Geometry: final body of the model. Coordinates: model frame, mm. Give positions to 0.01 mm unless a question says otherwise; leave off trailing zeros. Write each loop counter-clockwise with the first axis right and the second up, starting at its lowest first coordinate (ties: lowest second). Pieces come first, ordered by that corner, then holes.
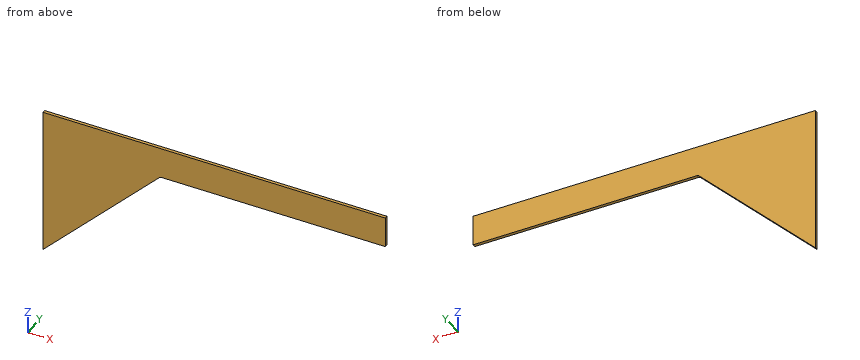
from build123d import *

# Parameters (mm, degrees)
BOSS_EXTRUDE1_DEPTH = 3.175
FILLET1_R           = 2.54


with BuildPart() as part:
    # Sketch1 → Boss-Extrude1 (new body)
    with BuildSketch(Plane(origin=(0, 0, 0), x_dir=(1, 0, 0), z_dir=(0, 1, 0))):
        Polygon((152.4, 0), (0, 0), (0, 152.4), align=None)
        Polygon((120.65, 31.75), (152.4, 0), (352.425, 0), (352.425, 31.75), (121.965128061, 31.75), align=None)
    extrude(amount=BOSS_EXTRUDE1_DEPTH)

    # Fillet1
    fillet1_edges = [part.edges().sort_by_distance(p)[0] for p in [
        (120.65, 1.5875, -31.75),
    ]]
    fillet(fillet1_edges, radius=FILLET1_R)


solid = part.part
Q1. Ray query, line 1 along Z through (x, y) = (336, 1.4); line 2 along X through (y, z) = (0.85, -104); line 3 along Z through (x, y) = (77, 1.7). Return the intervals inside material, ascending.
Filled sheet:
line 1: z = -31.75 to 0
line 2: x = 0 to 48.4
line 3: z = -75.4 to 0
Q2. Section C-C on z = -105. Output: boundary loops of the cut face in (x, y) (3 decimals).
Filled sheet:
outline: (0, 0) - (47.4, 0) - (47.4, 3.175) - (0, 3.175) - close
Q3. Section B-B on x = 90. Output: boundary loops of the cut face in (y, z) (3 decimals).
Filled sheet:
outline: (0, -62.4) - (3.175, -62.4) - (3.175, 0) - (0, 0) - close
Q4. Section A-A on y = 0.7. Output: boundary loops of the cut face in (x, z) (3 decimals).
Filled sheet:
outline: (0, -152.4) - (119.906, -32.494) arc R2.54 cw to (121.702, -31.75) - (352.425, -31.75) - (352.425, 0) - (0, 0) - close
Q5. Pin query (flat end, axial travel): P1, Ø1.5, axis at x = 48, y = 2.5, coming from the -Z side. Return the tip coordinate at first contact, or that it passes through.
Filled sheet:
P1: stops at z = -105.15
